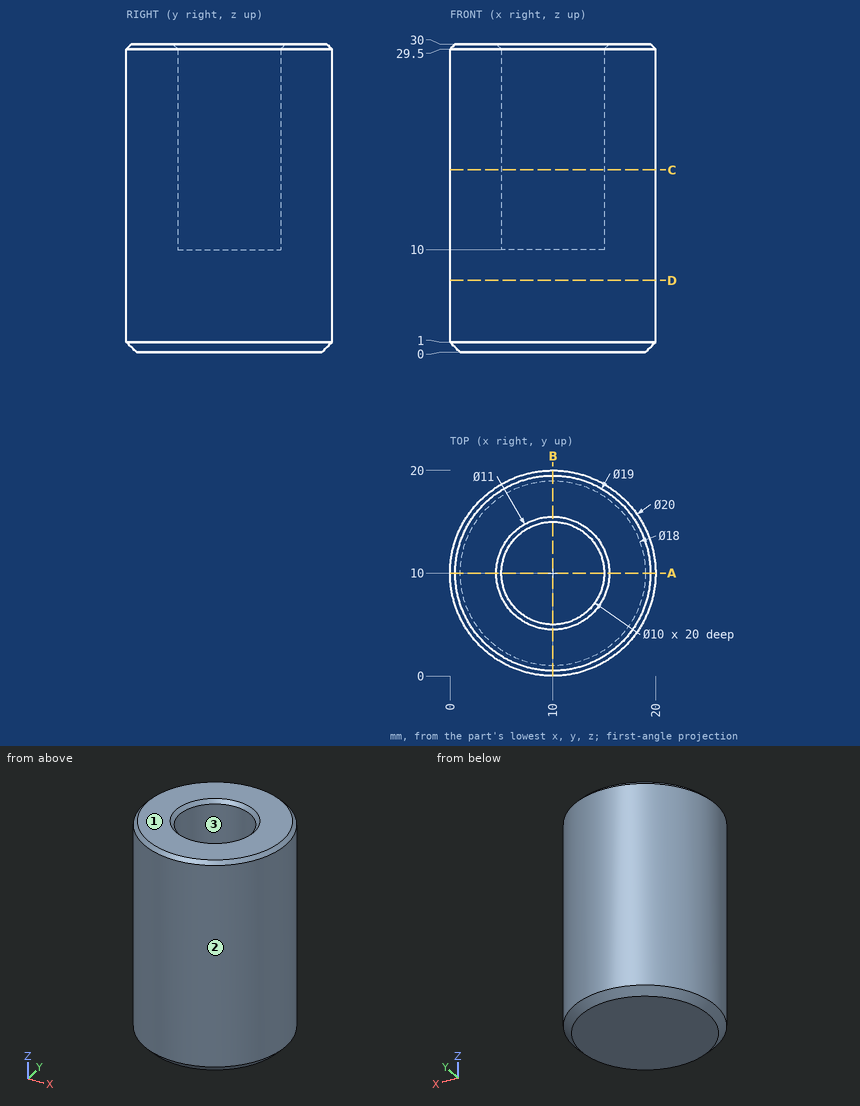
Input: dimensioned drawing with shaded views. Units: mm. Origin: part minimum x, y, z. Round coordinates to 2 decimals unless told otherwise and drop trailing zeros. Loops run counter-clockwise (first coordinate to the right, second up) from the corner with the lowest first, then second, coordinate; pieces in that order, holes last. Notation, with made-up numbers: M -4,41.25 L 33,41.25 A32 cw 33,71.25 Z; hole C 79.25,71 d10. An arc over 180 degrees is marked long. Answer in a Markdown table with one row per item. Add a question column.
1. Section A-A (y = 10). Output: boundary loops of the cut face in (x, z).
2. Section C-C (z = 17.75). Output: boundary loops of the cut face in (x, y), and give its area (3 significant figures).
3. Ray query, probe 1 along X at (y, z) = (10, 19); probe 2 along Z at (x, y) = (9.5, 12.25). Return the intervals inside material, ascending.
4. Mould query, pull axis X, two halves, no side actions, for the marked faces 1, 2 and 3. Classes: released by +X, released by -X, zero draft, split by the parting line, or undercut.
5. Section D-D (z = 7). Output: boundary loops of the cut face in (x, y), and give its area (3 significant figures).
6. Contact query for flat-ended pins moving along their axis: pin 1 (3 mm diameter, centred on x = 3.5, y = 13.5, fed in from -Z); pin 2 (8 mm diameter, centred on y = 5, z = 8.5, fed in from -X); pin 3 (4 mm diameter, centred on x = 7.5, z = 6, fed in from -Y); pin 4 (2 mm diameter, centred on x = 3, z = 8.5, fed in from -Y). Output: stop coordinate, or through.
Values follow:
| question | item | result |
|---|---|---|
| 1 | outline | M 0,1 L 1,0 L 19,0 L 20,1 L 20,29.5 L 19.5,30 L 15.5,30 L 15,29.5 L 15,10 L 5,10 L 5,29.5 L 4.5,30 L 0.5,30 L 0,29.5 Z |
| 2 | outline | C 10,10 d20; hole C 10,10 d10 |
| 2 | area | 236 mm^2 |
| 3 | probe 1 | 0 to 5, 15 to 20 |
| 3 | probe 2 | 0 to 10 |
| 4 | face 1 | zero draft |
| 4 | face 2 | split by the parting line |
| 4 | face 3 | undercut |
| 5 | outline | C 10,10 d20 |
| 5 | area | 314 mm^2 |
| 6 | pin 1 | z = 0 |
| 6 | pin 2 | x = 0.05 |
| 6 | pin 3 | y = 0.01 |
| 6 | pin 4 | y = 2 |
